The drawing under review shows one solid part. Ordinate dimensions are in mm from its lowest x, y, z. Round coordinates to 2 decimals unless told otherwise and drop trailing zeros. Order: outer loops, then holes, each group sorted by start corner. A loop starts at its lowest first (then second) coordinate and runs counter-clockwise, first axis right, second up. Notation, with made-up numbers: (42, 65.5) -> (80, 65.5) arc R9 ccw to (80, 73.5) -> close; hole circle Ø1 at (-37, -35.5). An arc over 180 degrees is marked (long way). Use a Markdown table: item, result. Add a question column.
1) Consider section C-C (x = 25). State the section outline as (y, z) points, plus the area to 3 significant figures.
2) Wall thickness on line 1 along X through (y, z) = (0.65, 24); line 2 along X through (y, z) = (11.5, 14.25); line 3 along Y through (x, z) = (41, 10.5): over which ranges is each line inside the solid? List them lowest first. Write a range as [from, to].
3) Draft analysis for pull direction Y (two halves, no side actions). For the marked faces 1, 2 and 3, state which applies: pulls with the +Y half, pulls with the -Y half, needs draft (parallel to the pull), parting line crosses it, or undercut.
4) Consider section B-B (z = 18). State the section outline as (x, y) points.
5) Clearance check with flat-ended pins moving along their axes: P1, Ø7.5, axis at x = 5.5, y = 12, coming from the -Z side; P2, Ø5.5, axis at x = 34, z = 24, coming from the +Y side; P3, Ø7, axis at x = 16, z = 23.5, coming from the +Y side. State where each tip first meets the part, or that it passes through.
6) Consider section A-A (y = 11.5). State the section outline as (x, z) points.
7) Consider section D-D (z = 8.75). State the section outline as (x, y) points.
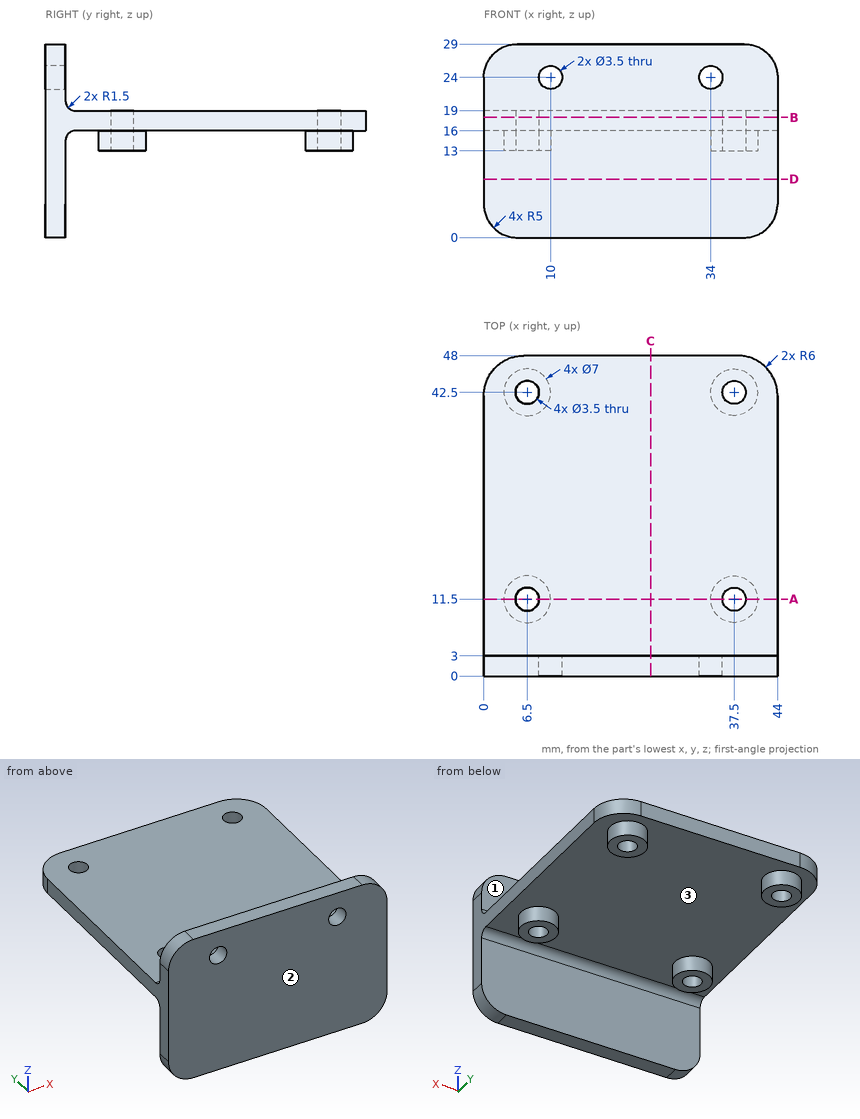
Results list:
| question | item | result |
|---|---|---|
| 1 | outline | (0, 0) -> (3, 0) -> (3, 14.5) arc R1.5 cw to (4.5, 16) -> (48, 16) -> (48, 19) -> (4.5, 19) arc R1.5 cw to (3, 20.5) -> (3, 29) -> (0, 29) -> close |
| 1 | area | 223 mm2 |
| 2 | line 1 | [0, 8.25], [11.75, 32.25], [35.75, 44] |
| 2 | line 2 | [3, 4.75], [8.25, 10], [34, 35.75], [39.25, 41] |
| 2 | line 3 | [0, 3] |
| 3 | face 1 | pulls with the +Y half |
| 3 | face 2 | pulls with the -Y half |
| 3 | face 3 | undercut |
| 4 | outline | (0, 0) -> (44, 0) -> (44, 42) arc R6 ccw to (38, 48) -> (6, 48) arc R6 ccw to (0, 42) -> close; hole circle Ø3.5 at (6.5, 11.5); hole circle Ø3.5 at (6.5, 42.5); hole circle Ø3.5 at (37.5, 11.5); hole circle Ø3.5 at (37.5, 42.5) |
| 5 | P1 | z = 13 |
| 5 | P2 | y = 3 |
| 5 | P3 | y = 3.09 |
| 6 | outline | (0, 16) -> (3, 16) -> (3, 13) -> (4.75, 13) -> (4.75, 19) -> (0, 19) -> close; (8.25, 13) -> (10, 13) -> (10, 16) -> (34, 16) -> (34, 13) -> (35.75, 13) -> (35.75, 19) -> (8.25, 19) -> close; (39.25, 13) -> (41, 13) -> (41, 16) -> (44, 16) -> (44, 19) -> (39.25, 19) -> close |
| 7 | outline | (0, 0) -> (44, 0) -> (44, 3) -> (0, 3) -> close |
